Design review of the part built by this model. Coordinates are the model's own, in mm. A direction names the side the tool comes from. Round coordinates to 2 decimals unless told otherwise and drop trailing zeros. Loops run counter-clockwise (first coordinate to the right, second up) from the corner with the lowest first, then second, coordinate; pieces in that order, holes last. Notation, with made-up numbers: (37.5, -3) -> (65.5, -3) arc R17 cw to (65.5, 27) -> close; hole circle Ø8 at (-22, 17). An arc over 180 degrees is marked (long way). Use a Markdown table: item, result. Add a question column.
Autodesk Fusion 360 part; units mm, degrees
sketch "Sketch1" plane through (0, 0, 0) normal (0, 0, 1) x (1, 0, 0)
  circle A0 centre (-76, 32) radius 1.6
  circle A1 centre (-31, 40) radius 1.6
  circle A2 centre (31, 40) radius 1.6
  circle A3 centre (76, 32) radius 1.6
  circle A4 centre (-76, -37) radius 1.6
  circle A5 centre (-24, -40) radius 1.6
  circle A6 centre (26, -40) radius 1.6
  circle A7 centre (76, -37) radius 1.6
  line L0 (-80, 44) -> (80, 44)
  line L1 (80, 44) -> (80, -44)
  line L2 (80, -44) -> (-80, -44)
  line L3 (-80, -44) -> (-80, 44)
  line L4 (80, 44) -> (-80, -44) construction
  dimension "d1" = 3.2
  dimension "d2" = 69
  dimension "d3" = 152
  dimension "d4" = 50
  dimension "d5" = 62
  dimension "d6" = 7
  dimension "d7" = 160
  dimension "d8" = 4
  dimension "d9" = 88
  dimension "d10" = 4
  dimension "d11" = 4
  dimension "d13" = 49
  dimension "d21" = 56
sketch "Sketch2" plane through (0, 0, 0) normal (0, 0, 1) x (1, 0, 0)
  circle A0 centre (-76, 32) radius 1.6 construction
  circle A1 centre (-31, 40) radius 1.6 construction
  circle A2 centre (31, 40) radius 1.6 construction
  circle A3 centre (76, 32) radius 1.6 construction
  circle A4 centre (76, -37) radius 1.6 construction
  circle A5 centre (26, -40) radius 1.6 construction
  circle A6 centre (-24, -40) radius 1.6 construction
  circle A7 centre (-76, -37) radius 1.6 construction
  circle A8 centre (-76, 32) radius 3 construction
  circle A9 centre (-31, 40) radius 3 construction
  circle A10 centre (31, 40) radius 3 construction
  circle A11 centre (76, 32) radius 3 construction
  circle A12 centre (76, -37) radius 3 construction
  circle A13 centre (26, -40) radius 3 construction
  circle A14 centre (-24, -40) radius 3 construction
  circle A15 centre (-76, -37) radius 3 construction
  line L0 (-79, 32) -> (-79, -37)
  arc A16 (-79, -37) -> (-73, -37) centre (-76, -37) ccw
  line L1 (-73, -37) -> (-73, 32)
  arc A17 (-73, 32) -> (-79, 32) centre (-76, 32) ccw
  line L2 (-76, 32) -> (-76, -37) construction
  line L3 (-76.1728, -39.995) -> (-24.1728, -42.995)
  arc A18 (-24.1728, -42.995) -> (-23.8272, -37.005) centre (-24, -40) ccw
  line L4 (-23.8272, -37.005) -> (-75.8272, -34.005)
  arc A19 (-75.8272, -34.005) -> (-76.1728, -39.995) centre (-76, -37) ccw
  line L5 (-76, -37) -> (-24, -40) construction
  line L6 (-75.4749, 29.0463) -> (-30.4749, 37.0463)
  arc A20 (-30.4749, 37.0463) -> (-31.5251, 42.9537) centre (-31, 40) ccw
  line L7 (-31.5251, 42.9537) -> (-76.5251, 34.9537)
  arc A21 (-76.5251, 34.9537) -> (-75.4749, 29.0463) centre (-76, 32) ccw
  line L8 (-76, 32) -> (-31, 40) construction
  line L9 (-31, 37) -> (31, 37)
  arc A22 (31, 37) -> (31, 43) centre (31, 40) ccw
  line L10 (31, 43) -> (-31, 43)
  arc A23 (-31, 43) -> (-31, 37) centre (-31, 40) ccw
  line L11 (-31, 40) -> (31, 40) construction
  line L12 (30.4749, 37.0463) -> (75.4749, 29.0463)
  arc A24 (75.4749, 29.0463) -> (76.5251, 34.9537) centre (76, 32) ccw
  line L13 (76.5251, 34.9537) -> (31.5251, 42.9537)
  arc A25 (31.5251, 42.9537) -> (30.4749, 37.0463) centre (31, 40) ccw
  line L14 (31, 40) -> (76, 32) construction
  line L15 (73, 32) -> (73, -37)
  arc A26 (73, -37) -> (79, -37) centre (76, -37) ccw
  line L16 (79, -37) -> (79, 32)
  arc A27 (79, 32) -> (73, 32) centre (76, 32) ccw
  line L17 (76, 32) -> (76, -37) construction
  line L18 (75.8203, -34.0054) -> (25.8203, -37.0054)
  arc A28 (25.8203, -37.0054) -> (26.1797, -42.9946) centre (26, -40) ccw
  line L19 (26.1797, -42.9946) -> (76.1797, -39.9946)
  arc A29 (76.1797, -39.9946) -> (75.8203, -34.0054) centre (76, -37) ccw
  line L20 (76, -37) -> (26, -40) construction
  line L21 (26, -37) -> (-24, -37)
  arc A30 (-24, -37) -> (-24, -43) centre (-24, -40) ccw
  line L22 (-24, -43) -> (26, -43)
  arc A31 (26, -43) -> (26, -37) centre (26, -40) ccw
  line L23 (26, -40) -> (-24, -40) construction
  dimension "d14" = 6
extrude "Extrude1" add sketch "Sketch2" along normal blind 6 contours L0 L1 L4 A19 L6 A21 | L1 A17 L6 A21 | A16 L1 L4 A19 | L1 A17 L6 L7 L9 A23 | A16 L1 L3 L4 L21 A30 | L6 A20 L9 A23 | A18 L4 L21 A30 | L6 A20 L9 L10 L12 A25 | A18 L4 L18 A28 L21 L22 | L9 A22 L12 A25 | L9 A22 L12 L13 L15 A27 | L18 A28 L21 A31 | L15 A26 L18 L19 L21 A31 | L12 A24 L15 A27 | L12 A24 L15 L16 L18 A29 | L15 A26 L18 A29
sketch "Sketch3" plane through (0, 0, 0) normal (0, 0, -1) x (1, 0, 0)
  circle A0 centre (-76, 37) radius 3
  circle A1 centre (-24, 40) radius 3
  circle A2 centre (26, 40) radius 3
  circle A3 centre (76, 37) radius 3
  circle A4 centre (76, -32) radius 3
  circle A5 centre (31, -40) radius 3
  circle A6 centre (-31, -40) radius 3
  circle A7 centre (-76, -32) radius 3
extrude "Extrude2" add sketch "Sketch3" against normal blind 12
hole "Hole1" at (76, 32, 0) at (31, 40, 0) at (-31, 40, 0) at (-76, 32, 0) at (-76, -37, 0) at (-24, -40, 0) at (26, -40, 0) at (76, -37, 0) direction (0, 0, 1) diameter 3.2 end through all
equation "d6 = 5.4 mm + ( ( 3.2 / 2 ) * 1 mm )"
equation "d8 = 2.4 mm + ( ( 3.2 / 2 ) * 1 mm )"
equation "d10 = 2.4 mm + ( ( 3.2 / 2 ) * 1 mm )"
equation "d11 = 2.4 mm + ( ( 3.2 / 2 ) * 1 mm )"
equation "d13 = 47.4 mm + ( ( 3.2 / 2 ) * 1 mm )"
equation "d21 = 54.4 mm + ( ( 3.2 / 2 ) * 1 mm )"
1. To check wall thickness, follow probe 1 along Y at (x, z) = (-76, 9.25); probe 2 along X at (y, z) = (40, 9); probe 3 along X at (y, z) = (27.5, 3.25). State the ranges of each line that lie inside material, in increasing order. Write a range as from..to.
2. Insertion check: P1, Ø2.5, axis at x = -76, y = -37, coming from the -Z side; P2, Ø4, axis at x = -54.5, z = 4.5, coming from the +Y side. Each pin has a flat end and moves straight along its axis. Give the tip position at first contact, or say it passes through.
3. Mouldability with a two-part tool opening along X and no side actions: class faces 1 (the face through (-29.7, 41.3, 12)), 2 (the face through (-76.07, 30.4, 6.08)), 3 (the face through (78.28, 33.95, 2.96)) as +X half, -X half, draft (parallel to the pull), parting line (faces both ways), or undercut.
4. Consider section C-C on z = 4.5. Give the number of separate pieces and of enclosed holes in the cut face, plus the area to 3 significant figures.
5. Consider section A-A on x = 16. State the section outline as (y, z) points.
6. For faces 4 (the face through (23.79, -42.03, 8.96)), 5 (the face through (73, -2, 3)), 6 (the face through (0, -38, 0)), list the 3-axis set-ups (+Z, -Z, +X, -X, +Y, -Y) from which the entire face can be reached by the end or side of a thin tool; tool diameter is ignored.
7. Consider section B-B on y = -5. State the section outline as (x, z) points, plus the area to 3 significant figures.
Verdict:
| question | item | result |
|---|---|---|
| 1 | probe 1 | y = -40..-38.6, -35.4..-34, 29..30.4, 33.6..35 |
| 1 | probe 2 | x = -34..-32.6, -29.4..-28, 28..29.4, 32.6..34 |
| 1 | probe 3 | x = -79..-73, 73..79 |
| 2 | P1 | passes through |
| 2 | P2 | stops at y = 39.22 |
| 3 | face 1 | draft |
| 3 | face 2 | undercut |
| 3 | face 3 | +X half |
| 4 | separate pieces | 1 |
| 4 | enclosed holes | 9 |
| 4 | area | 2,590 mm² |
| 5 | outline | (-43, 0) -> (-37, 0) -> (-37, 6) -> (-43, 6) -> close; (37, 0) -> (43, 0) -> (43, 6) -> (37, 6) -> close |
| 6 | face 4 | +Z |
| 6 | face 5 | +Z, -Z |
| 6 | face 6 | -Z, +X, -X, +Y, -Y |
| 7 | outline | (-79, 0) -> (-73, 0) -> (-73, 6) -> (-79, 6) -> close; (73, 0) -> (79, 0) -> (79, 6) -> (73, 6) -> close |
| 7 | area | 72.0 mm² |
